Part print with two shaded views. Sizes in mm from the minimum x, y, z corner. Round coordinates to 2 decimals unless told otherwise and drop trailing zeros. Order: outer loops, then holes, each group sorted by start corner. A loop starts at its lowest first (then second) coordinate and runs counter-clockwise, first axis right, second up. Notation, with made-up numbers: (15.25, 49.25) -> (39.25, 49.25) arc R31 cw to (39.25, 73.25) -> close; hole circle Ø11 at (78.25, -39.5). An arc over 180 degrees is marked (long way). Answer as a JSON object with one key per item and string values.
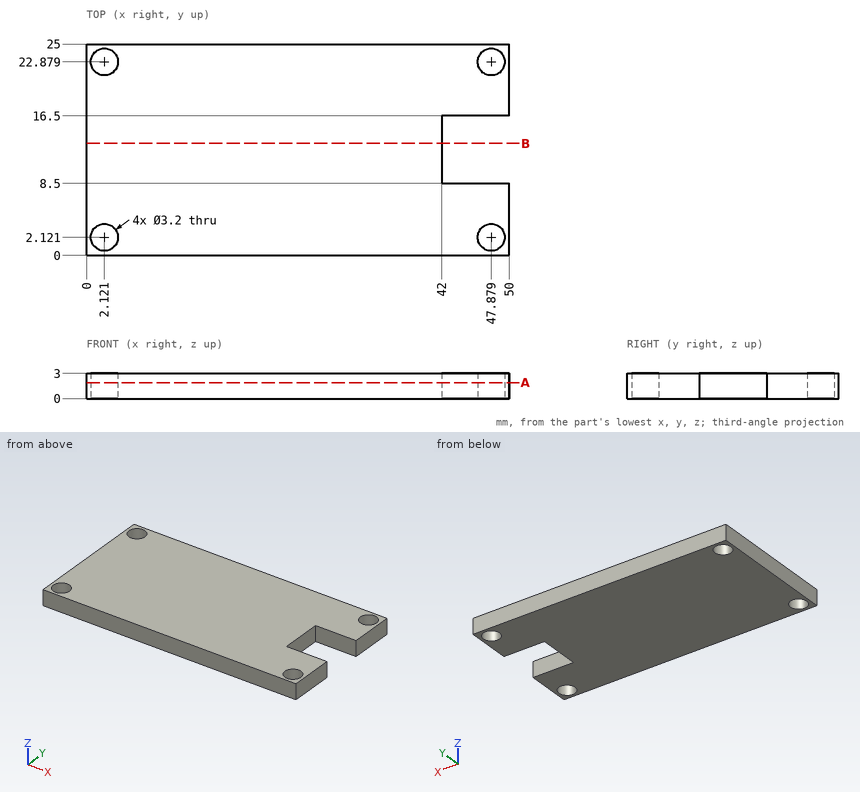
1) Cut at A-A, the plane z = 1.9. Give the cut face in (x, y).
Checked values:
{"outline": "(0, 0) -> (50, 0) -> (50, 8.5) -> (42, 8.5) -> (42, 16.5) -> (50, 16.5) -> (50, 25) -> (0, 25) -> close; hole circle Ø3.2 at (2.12, 2.12); hole circle Ø3.2 at (2.12, 22.88); hole circle Ø3.2 at (47.88, 2.12); hole circle Ø3.2 at (47.88, 22.88)"}
2) Probe L1, parallel to Y at x = 45, z = 0.35; L2, parallel to X at y = 2.5, z = 0.45 (1 decimal); L3, parallel to Y at x = 3, z = 2.3 (1 decimal). List the from-to ranges inside material, lowest first. Write a range as from..to.
Checked values:
{"L1": "y = 0..8.5, 16.5..25", "L2": "x = 0..0.6, 3.7..46.3, 49.4..50", "L3": "y = 0..0.8, 3.5..21.5, 24.2..25"}
3) Cut at B-B, the plane y = 13.25. Give the cut face in (x, z).
Checked values:
{"outline": "(0, 0) -> (42, 0) -> (42, 3) -> (0, 3) -> close"}
4) Flat gauge pin, fed straight in: pin 1 Ø4 at (x, y) = (2.12, 22.88) entering from +Z. Where does the tip first touch, or does it go through?
Checked values:
{"pin 1": "stops at z = 3"}
